```python
from build123d import *

# Parameters (mm, degrees)
SKETCH1_R           = 15.5
BOSS_EXTRUDE1_DEPTH = 4
SKETCH2_R           = 7
CENTER_HOLE_DEPTH   = 23.282279955
SKETCH3_R           = 1.5
M2_5_HOLE_DEPTH     = 23.282279955
CIRPATTERN1_COUNT   = 4


with BuildPart() as part:
    # Sketch1 → Boss-Extrude1 (new body)
    with BuildSketch(Plane(origin=(0, 0, 0), x_dir=(1, 0, 0), z_dir=(0, 1, 0))):
        with Locations(Location((0, 0, 0), (0, 0, 270))):
            Circle(SKETCH1_R)
    extrude(amount=BOSS_EXTRUDE1_DEPTH)

    # Sketch2 → center hole (cut, through all)
    with BuildSketch(Plane.XZ):
        with Locations(Location((0, 0, 0), (0, 0, 270))):
            Circle(SKETCH2_R)
    extrude(amount=-CENTER_HOLE_DEPTH, mode=Mode.SUBTRACT)

    # Sketch3 → M2.5 hole (cut, through all)
    with BuildSketch(Plane.XZ):
        with Locations(Location((0, 13, 0), (0, 0, 270))):
            Circle(SKETCH3_R)
    m2_5_hole = extrude(amount=-M2_5_HOLE_DEPTH, mode=Mode.SUBTRACT)

    # CirPattern1: M2.5 hole ×4 about axis
    cirpattern1_axis = Axis((0, 0, 0), (0, 1, 0))
    for i in range(1, CIRPATTERN1_COUNT):
        add(m2_5_hole.rotate(cirpattern1_axis, i * 360 / CIRPATTERN1_COUNT), mode=Mode.SUBTRACT)


solid = part.part
```
Source: CAD feature listing. Evaluate the final solid. Frame: model axes, mm. Give positions to 0.01 mm unless a question says otherwise; leave off trailing zeros. Order: outer loops, then holes, each group sorted by start corner. A loop starts at its lowest first (then second) coordinate and runs counter-clockwise, first axis right, second up.
(1) Section query D-D (x = 13). Return the cut outline in (y, z), plus the area to 3 significant figures.
(2) Section query A-A (z = 0). Return the cut outline in (x, y), plus the area to 3 significant figures.
(3) Material intervals for line 1 along Z through (x, y) = (1, 1.6); line 2 along X through (y, z) = (1.35, -3.5), sorted ascending.
(4) Section query B-B (x = 0). Return the cut outline in (y, z), plus the area to 3 significant figures.
(5) Section query C-C (z = -3.5). Return the cut outline in (x, y), plus the area to 3 significant figures.
(6) Contact query for flat-ended pins moving along their axis: P1, Ø2, axis at x = 11, y = 1, coming from the +Z side; P2, Ø1.5, axis at x = 11.5, y = 3.5, coming from the +Z side; P3, Ø1, axis at x = 4.5, y = 1.5, coming from the -Z side (3 decimals). Output: stop coordinate, or through.
(7) Pull-direction query (X, two-part tool) for faces 1 (the face through (14.5, 1.97, -0.07)), 2 (the face through (-3, 0, 7)), 3 (the face through (15.368, 1.972, -2.018)); classes: +X half, -X half, draft (parallel to the pull), parting line (faces both ways), or undercut.
Outcome:
1. outline: (0, -8.44) - (4, -8.44) - (4, -1.5) - (0, -1.5) - close; (0, 1.5) - (4, 1.5) - (4, 8.44) - (0, 8.44) - close
1. area: 55.5 mm2
2. outline: (-15.5, 0) - (-14.5, 0) - (-14.5, 4) - (-15.5, 4) - close; (-11.5, 0) - (-7, 0) - (-7, 4) - (-11.5, 4) - close; (7, 0) - (11.5, 0) - (11.5, 4) - (7, 4) - close; (14.5, 0) - (15.5, 0) - (15.5, 4) - (14.5, 4) - close
2. area: 44.0 mm2
3. line 1: z = -15.47 to -14.12, -11.88 to -6.93, 6.93 to 11.88, 14.12 to 15.47
3. line 2: x = -15.1 to -6.06, 6.06 to 15.1
4. outline: (0, -15.5) - (4, -15.5) - (4, -14.5) - (0, -14.5) - close; (0, -11.5) - (4, -11.5) - (4, -7) - (0, -7) - close; (0, 7) - (4, 7) - (4, 11.5) - (0, 11.5) - close; (0, 14.5) - (4, 14.5) - (4, 15.5) - (0, 15.5) - close
4. area: 44.0 mm2
5. outline: (-15.1, 0) - (-6.06, 0) - (-6.06, 4) - (-15.1, 4) - close; (6.06, 0) - (15.1, 0) - (15.1, 4) - (6.06, 4) - close
5. area: 72.3 mm2
6. P1: stops at z = 11.84
6. P2: stops at z = 11.17
6. P3: stops at z = -14.975
7. face 1: undercut
7. face 2: draft
7. face 3: parting line
